```python
from build123d import *

# Parameters (mm, degrees)
SKETCH1_R               = 34
BOSS_EXTRUDE1_DEPTH     = 48
CUT_EXTRUDE1_DEPTH      = 68.941151006
CUT_EXTRUDE1_DEPTH_BACK = 68.941151006
FILLET6_R               = 5
CUT_EXTRUDE2_DEPTH      = 82.215762187
CUT_EXTRUDE2_DEPTH_BACK = 82.215762187
SKETCH5_R               = 4.25
SKETCH6_R               = 9.55
CUT_EXTRUDE3_DEPTH      = 6.2
SKETCH7_R               = 4
BOSS_EXTRUDE2_DEPTH     = 5.5


with BuildPart() as part:
    # Sketch1 → Boss-Extrude1 (new body)
    with BuildSketch(Plane(origin=(0, 0, 0), x_dir=(1, 0, 0), z_dir=(0, 1, 0))):
        with Locations(Location((0, 0, 0), (0, 0, 270))):
            Circle(SKETCH1_R)
    extrude(amount=BOSS_EXTRUDE1_DEPTH)

    # Sketch3 → Cut-Extrude1 (cut, two sides: drawn at the far end of the back side and taken through both)
    with BuildSketch(Plane.XY.offset(-CUT_EXTRUDE1_DEPTH_BACK)):
        with BuildLine():
            Line((-22, -157.512711317), (-22, 0))
            Line((-22, 0), (-22, 24))
            ThreePointArc((-22, 24), (-19.071067812, 31.071067812), (-12, 34))
            Line((-12, 34), (12, 34))
            ThreePointArc((12, 34), (19.071067812, 31.071067812), (22, 24))
            Line((22, 24), (22, 0))
            Line((22, 0), (22, -157.512711317))
            Line((22, -157.512711317), (22, -472.53813395))
            Line((22, -472.53813395), (-22, -472.53813395))
            Line((-22, -472.53813395), (-22, -157.512711317))
        make_face()
    extrude(amount=CUT_EXTRUDE1_DEPTH + CUT_EXTRUDE1_DEPTH_BACK, mode=Mode.SUBTRACT)

    # Fillet6
    fillet6_edges = [part.edges().sort_by_distance(p)[0] for p in [
        (34, 0, 0),
        (-34, 0, 0),
        (-22, 0, 0),
        (22, 0, 0),
    ]]
    fillet(fillet6_edges, radius=FILLET6_R)

    # Sketch5 → Cut-Extrude2 (cut, two sides: drawn at the far end of the back side and taken through both)
    with BuildSketch(Plane(origin=(-22, 0, 0), x_dir=(0, 0, -1), z_dir=(1, 0, 0)).offset(-CUT_EXTRUDE2_DEPTH_BACK)):
        with Locations(Location((0, 14, 0), (0, 0, 90))):
            Circle(SKETCH5_R)
    extrude(amount=CUT_EXTRUDE2_DEPTH + CUT_EXTRUDE2_DEPTH_BACK, mode=Mode.SUBTRACT)

    # Sketch6 → Cut-Extrude3 (cut)
    with BuildSketch(Plane(origin=(-22, 0, 0), x_dir=(0, 0, -1), z_dir=(1, 0, 0))):
        with Locations(Location((0, 14, 0), (0, 0, 90))):
            Circle(SKETCH6_R)
    extrude(amount=-CUT_EXTRUDE3_DEPTH, mode=Mode.SUBTRACT)

    # Sketch7 → Boss-Extrude2 (add)
    with BuildSketch(Plane(origin=(0, 48, 0), x_dir=(1, 0, 0), z_dir=(0, 1, 0))):
        with Locations(Location((0, 0, 0), (0, 0, 270))):
            Circle(SKETCH7_R)
    extrude(amount=BOSS_EXTRUDE2_DEPTH)


solid = part.part
```
Part model, mm, in its own coordinate system. A direction names the side the tool comes from. Round coordinates to 2 decimals unless told otherwise and drop trailing zeros. Write each loop counter-clockwise with the first axis right and the second up, starting at its lowest first coordinate (ties: lowest second). Pieces come first, ordered by that corner, then holes. Notation, with made-up numbers: M 57,-34.5 L 63,-34.5 A34 ccw 63,-3.5 Z; hole C 65.5,54.5 d2. An arc over 180 degrees is marked long. Answer as CSV lines item,"result". Start each with the question number.
1) Band-saw the part on D-D (y = 27). List the corners of the cut face in (x, z), then the cut area to 3 significant figures.
2) Band-saw the part on C-C (z = 0). Count the separate pieces of the cut face and the enclosed holes in it, then the cut area to 3 significant figures.
3) Band-saw the part on A-A (x = 0). List the corners of the cut face in (y, z), then the cut area to 3 significant figures.
4) Drill centre lines: L1, parallel to Y at x = 28.5, z = 0; L2, parallel to X at y = 18, z = -22; L3, parallel to Y at x = -11.5, z = -3. Where is each one in solid material? Low to high.
5) Band-saw the part on B-B (y = 14). List the corners of the cut face in (x, z), then the cut area to 3 significant figures.
6) Mould opens along X. For faces 1 (the face through (-25.06, 22.82, -3.66)), 2 (the face through (0, 34, 0)), 3 (the face through (-3.905, 50.712, -0.867)), 4 (the face through (-31.145, 17.926, -1.628)) say: +X half, -X half, draft (parallel to the pull), parting line (faces both ways), or undercut.
7) Which spindle directions (+Z, -Z, +X, -X, +Y, -Y) get a long thin tool onto all of the face, cutting with end or side? Do faces 5 (the face through (28, 0, 0)), 6 (the face through (-28.2, 16, -4)), 7 (the face through (22, 19, 0)). Say none if no direction does.
8) Drop flat-ended pins along their axis: pin 1 (8 mm diameter, centred on y = 42.5, z = 5, fed in from -X); pin 2 (11 mm diameter, centred on y = 14, z = 0, fed in from +X); pin 3 (1.5 mm diameter, centred on y = 13.5, z = -15, fed in from +X); pin 4 (8 mm diameter, centred on x = -27, y = 24.5, fed in from -Z). Give the stop position or say it passes through.
Worked out:
1,outline,"M -21.54,-26.31 L -21.54,26.31 A34 ccw Z; M 21.54,-26.31 A34 ccw 21.54,26.31 Z"
1,area,"912 mm²"
2,separate pieces,"3"
2,enclosed holes,"0"
2,area,"1,560 mm²"
3,outline,"M 34,-34 L 48,-34 L 48,-4 L 53.5,-4 L 53.5,4 L 48,4 L 48,34 L 34,34 Z"
3,area,"996 mm²"
4,L1,"0 to 9.75, 18.25 to 48"
4,L2,"-25.92 to -22, 22 to 25.92"
4,L3,"34 to 48"
5,outline,"M -33.73,-4.25 A34 ccw -22,-25.92 L -22,-9.55 L -28.2,-9.55 L -28.2,-4.25 Z; M -33.73,4.25 L -28.2,4.25 L -28.2,9.55 L -22,9.55 L -22,25.92 A34 ccw Z; M 22,-25.92 A34 ccw 33.73,-4.25 L 22,-4.25 Z; M 22,4.25 L 33.73,4.25 A34 ccw 22,25.92 Z"
5,area,"596 mm²"
6,face 1,"undercut"
6,face 2,"undercut"
6,face 3,"parting line"
6,face 4,"draft"
7,face 5,"+Z, -Z, +X, -X, -Y"
7,face 6,"none"
7,face 7,"+Z, -Z, -Y"
8,pin 1,"x = -33.99"
8,pin 2,"x = 34"
8,pin 3,"x = 30.87"
8,pin 4,"z = -25.04"
